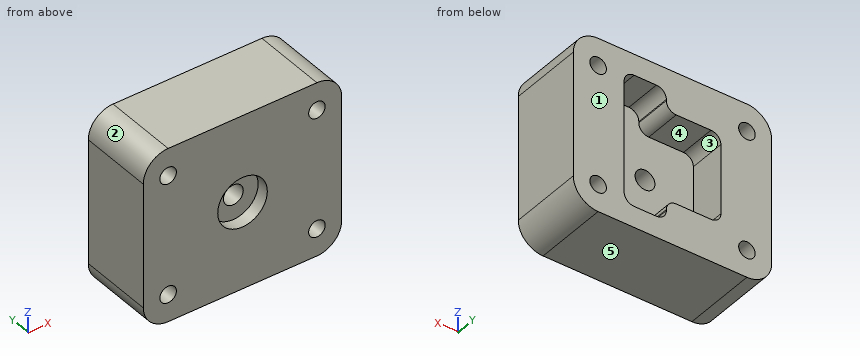
from build123d import *

# Parameters (mm, degrees)
SKETCH1_W           = 40
SKETCH1_H           = 35
SKETCH1_R           = 1.666666667
BOSS_EXTRUDE1_DEPTH = 15
FILLET1_R           = 5
CUT_EXTRUDE1_DEPTH  = 7.5
FILLET2_R           = 2
SKETCH5_R           = 2
CUT_EXTRUDE2_DEPTH  = 7.5
SKETCH6_R           = 5
CUT_EXTRUDE3_DEPTH  = 2.5


with BuildPart() as part:
    # Sketch1 → Boss-Extrude1 (new body)
    with BuildSketch(Plane(origin=(0, 0, 0), x_dir=(1, 0, 0), z_dir=(0, 1, 0))):
        with Locations((20, 17.5)):
            Rectangle(SKETCH1_W, SKETCH1_H)
        with Locations(Location((5, 29.5, 0), (0, 0, 270))):
            Circle(SKETCH1_R, mode=Mode.SUBTRACT)
        with Locations(Location((35, 29.5, 0), (0, 0, 270))):
            Circle(SKETCH1_R, mode=Mode.SUBTRACT)
        with Locations(Location((5, 5.5, 0), (0, 0, 270))):
            Circle(SKETCH1_R, mode=Mode.SUBTRACT)
        with Locations(Location((35, 5.5, 0), (0, 0, 270))):
            Circle(SKETCH1_R, mode=Mode.SUBTRACT)
    extrude(amount=BOSS_EXTRUDE1_DEPTH)

    # Fillet1
    fillet1_edges = [part.edges().sort_by_distance(p)[0] for p in [
        (0, 7.5, -35),
        (40, 7.5, -35),
        (40, 7.5, 0),
        (0, 7.5, 0),
    ]]
    fillet(fillet1_edges, radius=FILLET1_R)

    # Sketch4 → Cut-Extrude1 (cut)
    with BuildSketch(Plane(origin=(0, 15, 0), x_dir=(1, 0, 0), z_dir=(0, 1, 0))):
        Polygon((29.75, 30.75), (21.25, 30.75), (21.25, 26.5), (10.25, 26.5), (10.25, 8.5), (21.25, 8.5), (21.25, 4.25), (29.75, 4.25), align=None)
    extrude(amount=-CUT_EXTRUDE1_DEPTH, mode=Mode.SUBTRACT)

    # Fillet2
    fillet2_edges = [part.edges().sort_by_distance(p)[0] for p in [
        (21.25, 11.25, -26.5),
        (21.25, 11.25, -30.75),
        (29.75, 11.25, -30.75),
        (29.75, 11.25, -4.25),
        (21.25, 11.25, -4.25),
        (21.25, 11.25, -8.5),
        (10.25, 11.25, -8.5),
        (10.25, 11.25, -26.5),
    ]]
    fillet(fillet2_edges, radius=FILLET2_R)

    # Sketch5 → Cut-Extrude2 (cut)
    with BuildSketch(Plane(origin=(0, 7.5, 0), x_dir=(1, 0, 0), z_dir=(0, 1, 0))):
        with Locations(Location((20, 17.5, 0), (0, 0, 270))):
            Circle(SKETCH5_R)
    extrude(amount=-CUT_EXTRUDE2_DEPTH, mode=Mode.SUBTRACT)

    # Sketch6 → Cut-Extrude3 (cut)
    with BuildSketch(Plane.XZ):
        with Locations(Location((20, -17.5, 0), (0, 0, 270))):
            Circle(SKETCH6_R)
    extrude(amount=-CUT_EXTRUDE3_DEPTH, mode=Mode.SUBTRACT)


solid = part.part
Verification items for the finished model (mm, model axes). Face numbers are marked on the shaded views. A direction names the side the tool comes from. Coordinates: 2 decimals unless noted, no trailing zeros. Order: outer loops, then holes, each group sorted by start corner. A loop starts at its lowest first (then second) coordinate and runs counter-clockwise, first axis right, second up. Notation, with made-up numbers: (-7.75, -10) -> (21.25, -10) arc R10 cw to (21.25, 7) -> close; hole circle Ø9 at (23.5, 46). An arc over 180 degrees is marked (long way). Use CSV: the item, a comma, the result in double quotes. Start each with the question number.
Q1. Section check A-A, the plane y = 9.5. Record the cut outline in (x, z), and give its area (3 significant figures).
Q2. Draft check along Z on the marked faces 1, 2 and 3. Enter one of: +Z half, -Z half, draft (parallel to the pull), parting line (faces both ways), or undercut.
Q3. Section check C-C, the plane x = 20. Record the cut outline in (y, z), and give its area (3 significant figures).
Q4. Section check D-D, the plane z = -5.5. Record the cut outline in (x, y), and give its area (3 significant figures).
Q5. Thickness scan on line 1 along X through (y, z) = (6, -29.5); line 2 along X through (y, z) = (6.05, -17.5); line 3 along X through (y, z) = (13, -20). Record the ranges inside material, lowest first.
Q6. Tool access check on the marked faces 4 and 5. Record the directions out of +Z, -Z, +X, -X, +Y, -Y that give a thin tool (end or side, any length) a straight path to the whole face; none if there is none.
Q7. Section check B-B, the plane z = -17.5. Record the cut outline in (x, y).
Q8. Depth check by flat-ended pin: P1, Ø3, axis at x = 20.5, z = -19, coming from the -Y side; P2, Ø2, axis at x = 35, z = -5.5, coming from the +Y side; P3, Ø6, axis at x = 24.5, z = -15, coming from the +Y side. Enter the tip coordinate at first touch or a pass-through.
Returned:
1,outline,"(0, -30) arc R5 ccw to (5, -35) -> (35, -35) arc R5 ccw to (40, -30) -> (40, -5) arc R5 ccw to (35, 0) -> (5, 0) arc R5 ccw to (0, -5) -> close; hole circle Ø3.33 at (5, -29.5); hole circle Ø3.33 at (5, -5.5); hole (10.25, -24.5) arc R2 ccw to (12.25, -26.5) -> (19.25, -26.5) arc R2 cw to (21.25, -28.5) -> (21.25, -28.75) arc R2 ccw to (23.25, -30.75) -> (27.75, -30.75) arc R2 ccw to (29.75, -28.75) -> (29.75, -6.25) arc R2 ccw to (27.75, -4.25) -> (23.25, -4.25) arc R2 ccw to (21.25, -6.25) -> (21.25, -6.5) arc R2 cw to (19.25, -8.5) -> (12.25, -8.5) arc R2 ccw to (10.25, -10.5) -> close; hole circle Ø3.33 at (35, -29.5); hole circle Ø3.33 at (35, -5.5)"
1,area,"924 mm^2"
2,face 1,"draft"
2,face 2,"+Z half"
2,face 3,"undercut"
3,outline,"(0, -35) -> (15, -35) -> (15, -26.65) -> (7.5, -26.65) -> (7.5, -19.5) -> (2.5, -19.5) -> (2.5, -22.5) -> (0, -22.5) -> close; (0, -12.5) -> (2.5, -12.5) -> (2.5, -15.5) -> (7.5, -15.5) -> (7.5, -8.35) -> (15, -8.35) -> (15, 0) -> (0, 0) -> close"
3,area,"343 mm^2"
4,outline,"(0, 0) -> (3.33, 0) -> (3.33, 15) -> (0, 15) -> close; (6.67, 0) -> (33.33, 0) -> (33.33, 15) -> (29.6, 15) -> (29.6, 7.5) -> (21.4, 7.5) -> (21.4, 15) -> (6.67, 15) -> close; (36.67, 0) -> (40, 0) -> (40, 15) -> (36.67, 15) -> close"
4,area,"438 mm^2"
5,line 1,"x = 0 to 3.33, 6.67 to 33.33, 36.67 to 40"
5,line 2,"x = 0 to 18, 22 to 40"
5,line 3,"x = 0 to 10.25, 29.75 to 40"
6,face 4,"+Y"
6,face 5,"-Z, +X, -X, +Y, -Y"
7,outline,"(0, 0) -> (15, 0) -> (15, 2.5) -> (18, 2.5) -> (18, 7.5) -> (10.25, 7.5) -> (10.25, 15) -> (0, 15) -> close; (22, 2.5) -> (25, 2.5) -> (25, 0) -> (40, 0) -> (40, 15) -> (29.75, 15) -> (29.75, 7.5) -> (22, 7.5) -> close"
8,P1,"stops at y = 2.5"
8,P2,"passes through"
8,P3,"stops at y = 7.5"
